Could you check a few things on this model? Use its own coordinates, in mm. Face numbers are marked on the shaded views. A direction names the side the tool comes from. Coordinates: 2 decimals unless noted, no trailing zeros. Write each loop counter-clockwise with the first axis right and the second up, starting at its lowest first coordinate (ties: lowest second). Pieces come first, ordered by that corner, then holes. Notation, with made-up numbers: (-18, 19.25) - (6, 19.25) arc R24 cw to (6, 31.25) - close; hole circle Ø9 at (74, 16). An arc over 180 degrees is marked (long way). Answer as a JSON object with one key per item and string values. Group by question number.
1) On a 3-axis mill with a long thin cutter (end or side, diameter ignored), from which of +Z, -Z, +X, -X, +Y, -Y can I reach the whole of each face in a straight line? I mean the marked faces 1 and 2. Say none if no direction works.
2) If we section it at A-A (x = -21): Write out the boundary of the cut face in (y, z), plus the area to 3 significant figures.
3) Please list where these lines run through material, in increasing order: line 1 along Y through (x, z) = (-23.5, 1011.5); line 2 along Z through (x, y) = (20, -9.5); line 3 along Z through (x, y) = (-41.5, 35).
4) If we section it at C-C (z = 980): Write out the boundary of the cut face in (x, y), plus the area to 3 significant figures.
5) If we section it at B-B (y = -14.5): Write out the boundary of the cut face in (x, z).
6) Will these pins go through, and if not, where does the flat tip stop? pin 1 Ø1.5 at (x, z) = (35, 971) entering from -Y; pin 2 Ø1.5 at (x, z) = (-55, 1059.5) entering from -Y; pin 3 Ø15 at (x, y) = (14.5, -1.5) entering from -Z.
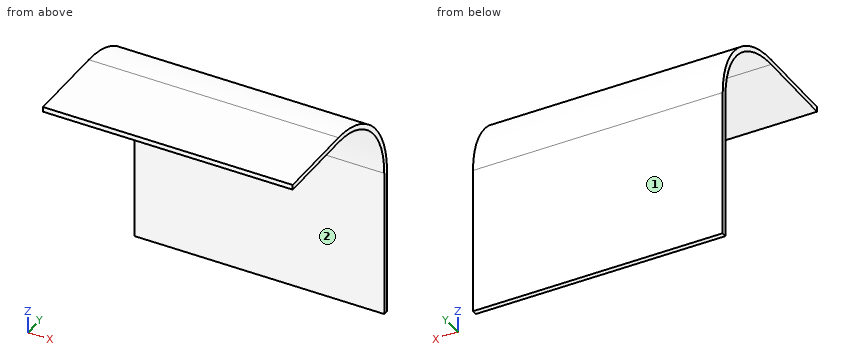
```python
from build123d import *

# Parameters (mm, degrees)
SALIENTE_EXTRUIR1_DEPTH = 75


with BuildPart() as part:
    # Croquis1 → Saliente-Extruir1 (new, symmetric)
    with BuildSketch(Plane(origin=(-7.305693887, -32.456719669, 940.926254751), x_dir=(0, 0, -1), z_dir=(1, 0, 0))):
        with BuildLine():
            Line((-90, 100), (0, 100))
            Line((0, 100), (0, 103))
            Line((0, 103), (-90, 103))
            ThreePointArc((-90, 103), (-127.476659403, 87.476659403), (-143, 50))
            Line((-143, 50), (-143, 0))
            Line((-143, 0), (-140, 0))
            Line((-140, 0), (-140, 50))
            ThreePointArc((-140, 50), (-125.355339059, 85.355339059), (-90, 100))
        make_face()
    extrude(amount=SALIENTE_EXTRUIR1_DEPTH, both=True)


solid = part.part
```
Here are the results:
{
 "1": {"face 1": "+Z, -Z, +X, -X, +Y", "face 2": "-Z, +X, -X, -Y"},
 "2": {"outline": "(-32.46, 1080.93) - (17.54, 1080.93) arc R50 cw to (67.54, 1030.93) - (67.54, 940.93) - (70.54, 940.93) - (70.54, 1030.93) arc R53 ccw to (17.54, 1083.93) - (-32.46, 1083.93) - close", "area": "663 mm²"},
 "3": {"line 1": "y = 67.54 to 70.54", "line 2": "z = 1080.93 to 1083.93", "line 3": "z = 1077.78 to 1080.97"},
 "4": {"outline": "(-82.31, 67.54) - (67.69, 67.54) - (67.69, 70.54) - (-82.31, 70.54) - close", "area": "450 mm²"},
 "5": {"outline": "(-82.31, 1080.93) - (67.69, 1080.93) - (67.69, 1083.93) - (-82.31, 1083.93) - close"},
 "6": {"pin 1": "stops at y = 67.54", "pin 2": "stops at y = 58.04", "pin 3": "stops at z = 1080.93"}
}
